Input: part model. Units: mm. Frame: model coordinates. A direction names the side the tool comes from. Coordinates: 2 decimals unless noted, no trailing zeros. Order: outer loops, then holes, each group sorted by start corner. A loop starts at its lowest first (then second) coordinate and runs counter-clockwise, first axis right, second up. Notation, with made-up numbers: (-7, 4) - (31, 4) arc R17 ccw to (31, 33) - close; hole circle Ø6 at (61, 29). An arc over 180 degrees is marked (long way). One line per question, with ' | ' between items.
from build123d import *

# Parameters (mm, degrees)
MOVE_BODY_2_DEPTH    = 3000
SKETCH_6_OUTSIDE_W   = 652.406
SKETCH_6_OUTSIDE_H   = 3602.406
SKETCH_6_OUTSIDE_W_2 = 50
SKETCH_6_OUTSIDE_H_2 = 899.25
CUT_EXTRUDE_1_DEPTH  = 3003.033019472


# Read off the part's stored shape, not the designer's step: Тело-Переместить/Копировать2
with BuildPart() as part:
    # Move Body 2 outline → Move Body 2 (new body)
    with BuildSketch(Plane(origin=(0, 0, 0), x_dir=(1, 0, 0), z_dir=(0, 1, 0))):
        with BuildLine():
            Line((-50, 47.75), (-50, 46.25))
            Line((-50, 46.25), (-49.25, 46.25))
            Line((-49.25, 46.25), (-49.25, 47.75))
            ThreePointArc((-49.25, 47.75), (-49.030330086, 48.280330086), (-48.5, 48.5))
            Line((-48.5, 48.5), (-1.5, 48.5))
            ThreePointArc((-1.5, 48.5), (-0.969669914, 48.280330086), (-0.75, 47.75))
            Line((-0.75, 47.75), (-0.75, -47.75))
            ThreePointArc((-0.75, -47.75), (-0.969669914, -48.280330086), (-1.5, -48.5))
            Line((-1.5, -48.5), (-48.5, -48.5))
            ThreePointArc((-48.5, -48.5), (-49.030330086, -48.280330086), (-49.25, -47.75))
            Line((-49.25, -47.75), (-49.25, -46.25))
            Line((-49.25, -46.25), (-50, -46.25))
            Line((-50, -46.25), (-50, -47.75))
            ThreePointArc((-50, -47.75), (-49.560660172, -48.810660172), (-48.5, -49.25))
            Line((-48.5, -49.25), (-1.5, -49.25))
            ThreePointArc((-1.5, -49.25), (-0.439339828, -48.810660172), (0, -47.75))
            Line((0, -47.75), (0, 47.75))
            ThreePointArc((0, 47.75), (-0.439339828, 48.810660172), (-1.5, 49.25))
            Line((-1.5, 49.25), (-48.5, 49.25))
            ThreePointArc((-48.5, 49.25), (-49.560660172, 48.810660172), (-50, 47.75))
        make_face()
    extrude(amount=MOVE_BODY_2_DEPTH)

    # Эскиз6 outside → Вырез-Вытянуть1 (cut, through all)
    with BuildSketch(Plane(origin=(0, 0, -49.25), x_dir=(-1, 0, 0), z_dir=(0, 0, -1))):
        with Locations((25, 1500)):
            Rectangle(SKETCH_6_OUTSIDE_W, SKETCH_6_OUTSIDE_H)
        with Locations((25, 449.625)):
            Rectangle(SKETCH_6_OUTSIDE_W_2, SKETCH_6_OUTSIDE_H_2, mode=Mode.SUBTRACT)
    extrude(amount=-CUT_EXTRUDE_1_DEPTH, mode=Mode.SUBTRACT)


solid = part.part
Item 1: Ray query, line 1 (Z direction, x = -40, y = 75.5); line 2 (X direction, y = 336, z = 36.5). Return the intervals inside material, ascending.
Data:
line 1: -49.25 to -48.5, 48.5 to 49.25 | line 2: -0.75 to 0
Item 2: Section C-C on z = -33.5. Return the cut outline in (x, y).
Data:
outline: (-0.75, 0) - (0, 0) - (0, 899.25) - (-0.75, 899.25) - close
Item 3: Contact query for flat-ended pins moving along their axis: P1, Ø0.6, axis at x = -49.5, y = 226.5, coming from the +Z side; P2, Ø0.6, axis at x = -49.5, y = 297.5, coming from the -Z side. Output: stop coordinate, or through.
Data:
P1: z = 49.08 | P2: z = -49.08
Item 4: Section B-B on y = 173.5. Return the cut outline in (x, z).
Data:
outline: (-50, -47.75) arc R1.5 ccw to (-48.5, -49.25) - (-1.5, -49.25) arc R1.5 ccw to (0, -47.75) - (0, 47.75) arc R1.5 ccw to (-1.5, 49.25) - (-48.5, 49.25) arc R1.5 ccw to (-50, 47.75) - (-50, 46.25) - (-49.25, 46.25) - (-49.25, 47.75) arc R0.75 cw to (-48.5, 48.5) - (-1.5, 48.5) arc R0.75 cw to (-0.75, 47.75) - (-0.75, -47.75) arc R0.75 cw to (-1.5, -48.5) - (-48.5, -48.5) arc R0.75 cw to (-49.25, -47.75) - (-49.25, -46.25) - (-50, -46.25) - close
Item 5: Draft query along X for faces 3 (the face through (-25, 443, -48.5)), 4 (the face through (0, 443, 1)), 5 (the face through (-25, 443, 49.25)). Return one class per face: released by +X, released by -X, zero draft, split by the parting line, or undercut.
Data:
face 3: undercut | face 4: released by +X | face 5: zero draft
Item 6: Section A-A on x = -32. Return the cut outline in (y, z), and give its area (3 significant figures).
Data:
outline: (0, -49.25) - (899.25, -49.25) - (899.25, -48.5) - (0, -48.5) - close; (0, 48.5) - (899.25, 48.5) - (899.25, 49.25) - (0, 49.25) - close | area: 1,350 mm^2
Item 7: Access query for faces 1 (the face through (-25, 443, -49.25)), 2 (the face through (-25, 443, 48.5)). Directions: +Z, -Z, +X, -X, +Y, -Y. A direction counts if a zero-diameter tool reaches every point of the face in a straight line with its end or side. Return the directions, or none.
Data:
face 1: -Z, +X, -X, +Y, -Y | face 2: +Y, -Y
